Job drawing, mm, ordinate dimensions from the low corner. One solid piece. Give positions to 0.01 mm unless a question says otherwise; leave off trailing zeros. Loops run counter-clockwise (first coordinate to the right, second up) from the corner with the lowest first, then second, coordinate; pieces in that order, holes last. Notation, with made-up numbers: (70, -27.75) - (101, -27.75) arc R30 ccw to (101, 3.25) - close; hole circle Ø6 at (-10, -38). An arc over 180 degrees is marked (long way). Use a Markdown table: item, result.
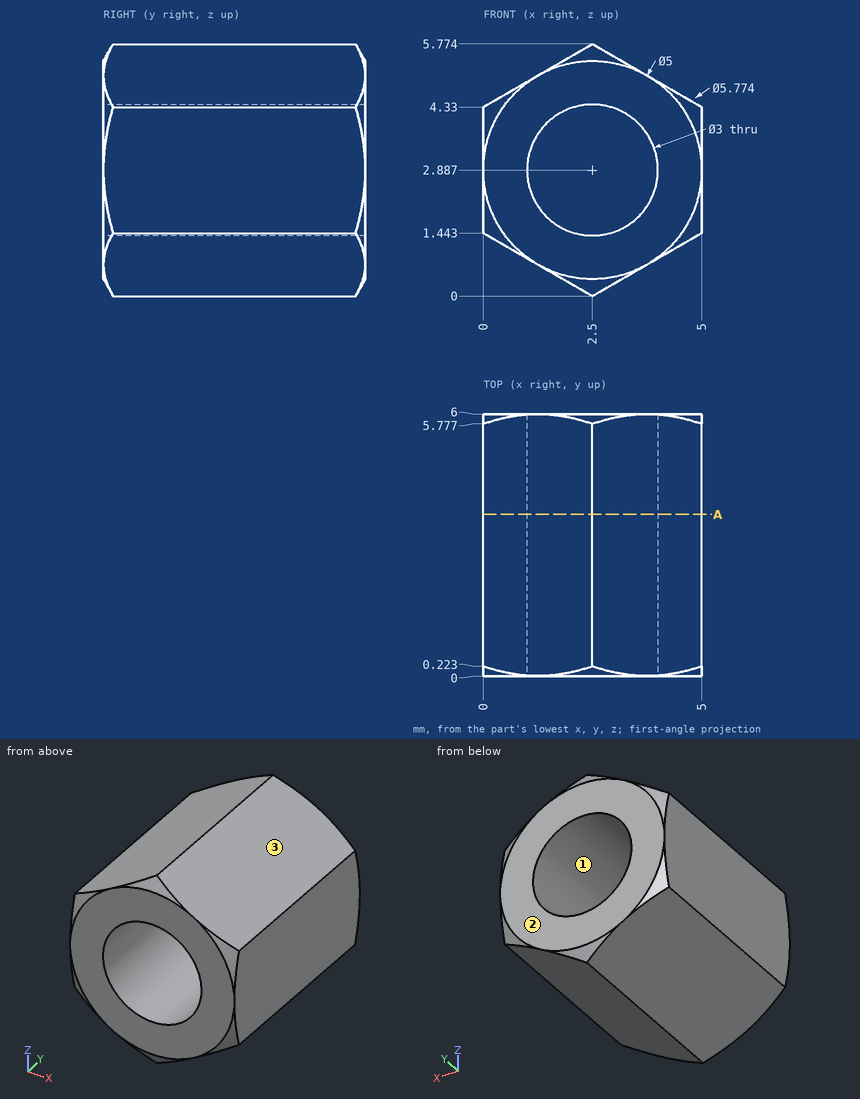
(1) Pin check, flat tips, straight feed: P1, Ø2, axis at y = 1.5, z = 1, coming from the -X side; P2, Ø3, axis at x = 2.5, y = 2, coming from the -Z side; P3, Ø1, axis at y = 4, z = 5, coming from the +X side (1 decimal). Stop position of each tip, or through.
Computed:
| item | result |
|---|---|
| P1 | x = 0 |
| P2 | z = 0 |
| P3 | x = 4.7 |
(2) Drill centre lines: probe 1 along X at (y, z) = (1.6, 2.5); probe 2 along Z at (x, y) = (1.3, 2.2) (1 decimal); probe 3 along Z at (x, y) = (2.35, 4.55) (1 decimal). Where is each one in solid material? Low to high. Write a range as [from, to].
Computed:
| item | result |
|---|---|
| probe 1 | [0, 1.05], [3.95, 5] |
| probe 2 | [0.7, 2], [3.8, 5.1] |
| probe 3 | [0.1, 1.4], [4.4, 5.7] |
(3) Slice it at A-A, the plane y = 3.7. Write the cut outline in (x, z).
Computed:
| item | result |
|---|---|
| outline | (0, 1.44) - (2.5, 0) - (5, 1.44) - (5, 4.33) - (2.5, 5.77) - (0, 4.33) - close; hole circle Ø3 at (2.5, 2.89) |
(4) Mould opens along X. For the marked faces 1, 2 and 3 say: pulls with the +X half, pulls with the -X half, needs draft (parallel to the pull), parting line crosses it, or undercut.
Computed:
| item | result |
|---|---|
| face 1 | undercut |
| face 2 | needs draft |
| face 3 | pulls with the +X half |
